from build123d import *

# Parameters (mm, degrees)
BOSS_EXTRUDE1_DEPTH = 3
SKETCH2_W           = 3
SKETCH2_H           = 19
BOSS_EXTRUDE2_DEPTH = 7
SKETCH3_W           = 1
SKETCH3_H           = 13
BOSS_EXTRUDE3_DEPTH = 2
SKETCH4_R           = 3.1
CUT_EXTRUDE2_DEPTH  = 3
SKETCH5_R           = 1.5
CUT_EXTRUDE3_DEPTH  = 3
FILLET1_R           = 1.5


with BuildPart() as part:
    # Sketch1 → Boss-Extrude1 (new body)
    with BuildSketch(Plane(origin=(0, -19, 0), x_dir=(1, 0, 0), z_dir=(0, 1, 0))):
        with BuildLine():
            Line((5.5, -7), (24, -7))
            Line((24, -7), (24, 7))
            Line((24, 7), (5.5, 7))
            ThreePointArc((5.5, 7), (-1.5, 0), (5.5, -7))
        make_face()
    extrude(amount=BOSS_EXTRUDE1_DEPTH)

    # Sketch2 → Boss-Extrude2 (add, symmetric)
    with BuildSketch(Plane.XY):
        with Locations((22.5, -9.5)):
            Rectangle(SKETCH2_W, SKETCH2_H)
    extrude(amount=BOSS_EXTRUDE2_DEPTH, both=True)

    # Sketch3 → Boss-Extrude3 (add)
    with BuildSketch(Plane(origin=(0, 0, 0), x_dir=(1, 0, 0), z_dir=(0, 1, 0))):
        with Locations((22.5, 0)):
            Rectangle(SKETCH3_W, SKETCH3_H)
    extrude(amount=BOSS_EXTRUDE3_DEPTH)

    # Sketch4 → Cut-Extrude2 (cut)
    with BuildSketch(Plane(origin=(0, -19, 0), x_dir=(1, 0, 0), z_dir=(0, 1, 0))):
        with Locations(Location((5.5, 0, 0), (0, 0, 270))):
            Circle(SKETCH4_R)
    extrude(amount=CUT_EXTRUDE2_DEPTH, mode=Mode.SUBTRACT)

    # Sketch5 → Cut-Extrude3 (cut)
    with BuildSketch(Plane(origin=(24, 0, 0), x_dir=(0, 0, -1), z_dir=(1, 0, 0))):
        with Locations((-4, -4)):
            Circle(SKETCH5_R)
        with Locations((4, -4)):
            Circle(SKETCH5_R)
    extrude(amount=-CUT_EXTRUDE3_DEPTH, mode=Mode.SUBTRACT)

    # Fillet1
    fillet1_edges = [part.edges().sort_by_distance(p)[0] for p in [
        (21, -16, 0),
    ]]
    fillet(fillet1_edges, radius=FILLET1_R)


solid = part.part
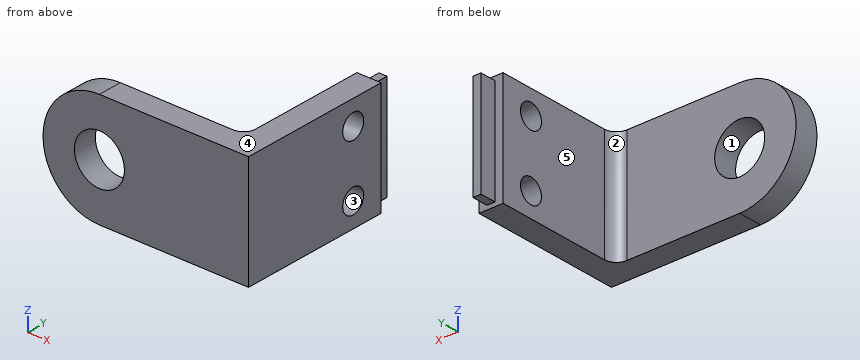
The listing builds one solid part. Answer for the finished solid, in the listing's coordinates (mm). Face numbers are marked on the shaded views. A direction names the side the tool comes from. Give positions to 0.01 mm unless a question says otherwise; leave off trailing zeros. Loops run counter-clockwise (first coordinate to the right, second up) from the corner with the lowest first, then second, coordinate; pieces in that order, holes last. Notation, with made-up numbers: (-6.75, 68) - (19.25, 68) arc R26 ccw to (19.25, 86) - close; hole circle Ø9 at (80.5, 80). An arc over 180 degrees is marked (long way). Write each question's results on one line, items separated by ' | '.
1. Flat-ended cylindrical pins translate along their axes: P1, Ø2, axis at y = 1.5, z = 1.5, coming from the -X side; P2, Ø1, axis at y = -6.5, z = -1.5, coming from the -X side; P3, Ø0.5, axis at x = 22.5, y = 1, coming from the +Z side; P4, Ø2.5, axis at y = -4, z = -4, coming from the +X side. Find the tip coordinate at first contact, or state that the pin passes through.
Resolved:
P1: stops at x = 22 | P2: stops at x = 21 | P3: stops at z = 6.5 | P4: passes through
2. For a pull along Y with two mould halves and no side action, classify the marked faces 1, 2 and 3 as +Y half, -Y half, draft (parallel to the pull), parting line (faces both ways), or undercut.
Resolved:
face 1: draft | face 2: +Y half | face 3: undercut
3. Find section D-D, the plane y = -16.5. Write down the section's boundary in (x, z).
Resolved:
outline: (5.5, -7) - (24, -7) - (24, 7) - (5.5, 7) arc R7 ccw to start; hole circle Ø6.2 at (5.5, 0)
4. Which of the six approach directions +Z, -Z, +X, -X, +Y, -Y give full straight-line access (tool end or side, diameter ignored) to the marked faces 4 and 5?
Resolved:
face 4: +Z, +X, -X, +Y, -Y | face 5: +Z, -Z, -X, +Y
5. Consider probe 1 along Y at (x, z) = (22.1, 4); probe 2 along X at (y, z) = (-16.7, 0); probe 3 along X at (y, z) = (-8.5, 2.5). Determine where each line is inside the solid, lowest interval first. Write a range as from..to.
Resolved:
probe 1: y = -19..-5.5, -2.5..2 | probe 2: x = -1.5..2.4, 8.6..24 | probe 3: x = 21..24
6. Find section A-A, the plane z = 0. Write down the section's boundary in (x, y).
Resolved:
outline: (-1.5, -19) - (2.4, -19) - (2.4, -16) - (-1.5, -16) - close; (8.6, -19) - (24, -19) - (24, 0) - (23, 0) - (23, 2) - (22, 2) - (22, 0) - (21, 0) - (21, -14.5) arc R1.5 cw to (19.5, -16) - (8.6, -16) - close
7. Find section C-C, the plane x = 6.75. Write down the section's boundary in (y, z), then the cut area to 3 significant figures.
Resolved:
outline: (-19, -7) - (-16, -7) - (-16, -2.84) - (-19, -2.84) - close; (-19, 2.84) - (-16, 2.84) - (-16, 7) - (-19, 7) - close | area: 25.0 mm^2
8. Find section B-B, the plane y = -4. Write down the section's boundary in (x, z), then the cut area to 3 significant figures.
Resolved:
outline: (21, -7) - (24, -7) - (24, -5.5) - (21, -5.5) - close; (21, -2.5) - (24, -2.5) - (24, 2.5) - (21, 2.5) - close; (21, 5.5) - (24, 5.5) - (24, 7) - (21, 7) - close | area: 24.0 mm^2
